from build123d import *

# Parameters (mm, degrees)
CHAMFER1_SIZE = 0.1


with BuildPart() as part:
    # Sketch1 → Revolve1 (revolve)
    with BuildSketch(Plane(origin=(0, 0, 0), x_dir=(0, 0, -1), z_dir=(1, 0, 0)), mode=Mode.PRIVATE) as revolve1_sk:
        Polygon((-3.5, 16), (3.5, 16), (3.5, 15.169361198), (3.160325371, 15.169361198), (3.160325371, 11.199592719), (3.5, 11.199592719), (3.5, 10), (-3.5, 10), (-3.5, 11.199592719), (-3.160325371, 11.199592719), (-3.160325371, 15.169361198), (-3.5, 15.169361198), align=None)
    revolve(revolve1_sk.sketch.rotate(Axis((0, 0, -19.078271996), (0, 0, 1)), 90), axis=Axis((0, 0, -19.078271996), (0, 0, 1)))

    # Chamfer1
    chamfer1_edges = [part.edges().sort_by_distance(p)[0] for p in [
        (15.169361198, 0, 3.5),
        (16, 0, 3.5),
        (16, 0, -3.5),
        (15.169361198, 0, -3.5),
        (11.199592719, 0, -3.5),
        (10, 0, -3.5),
        (10, 0, 3.5),
        (11.199592719, 0, 3.5),
    ]]
    chamfer(chamfer1_edges, length=CHAMFER1_SIZE)


solid = part.part
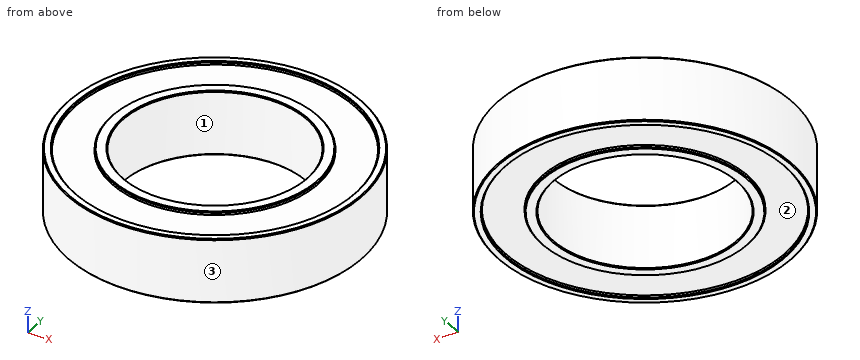
Verification items for the finished model (mm, model axes). Face numbers are marked on the shaded views. Give positions to 0.01 mm unless a question says otherwise; leave off trailing zeros. Order: outer loops, then holes, each group sorted by start corner. A loop starts at its lowest first (then second) coordinate and runs counter-clockwise, first axis right, second up. Notation, with made-up numbers: M 49,57 L 96,57 A26 cw 96,81 Z; hole C -4.75,70.5 d1. An arc over 180 degrees is marked long. Answer as a JSON object with one key per item and string values. Group by question number.
1) Mould release check, pull along Y, two halves, no side actions. Record for the marked faces 1, 2 and 3: released by +Y, released by -Y, zero draft, split by the parting line, or undercut.
2) Depth check by flat-ended pin: pin 1 Ø3 at (x, y) = (-6.5, -10) entering from -Z; pin 2 Ø1 at (x, z) = (-7.5, 1.5) entering from +Y; pin 3 Ø1.5 at (x, z) = (2, -2.5) entering from +Y. Enter the tip coordinate at first touch or a pass-through.
3) Cross-section at A-A (z = 0.5). Enter the section's corners in (x, y).
4) Scan lines: line 1 along Y through (x, z) = (0, -3.25); line 2 along Y through (x, z) = (0, 1.5); line 3 along Z through (x, y) = (14.5, 0.5). Record each from-to range of solid material in increasing order. Write a range as [from, to].
Result sheet:
{
 "1": {"face 1": "undercut", "face 2": "undercut", "face 3": "split by the parting line"},
 "2": {"pin 1": "stops at z = -3.5", "pin 2": "stops at y = 14.39", "pin 3": "stops at y = 15.95"},
 "3": {"outline": "C 0,0 d32; hole C 0,0 d20"},
 "4": {"line 1": "y = [-16, -15.17], [-11.2, -10], [10, 11.2], [15.17, 16]", "line 2": "y = [-16, -10], [10, 16]", "line 3": "z = [-3.16, 3.16]"}
}
